Work out the finished part from the listing and answer in its coordinate system (mm). A direction names the side the tool comes from. Give positions to 0.01 mm unless a question says otherwise; leave off trailing zeros. Write each loop counter-clockwise with the first axis right and the second up, starting at its lowest first coordinate (ties: lowest second). Pieces come first, ordered by that corner, then holes. Notation, with made-up numbers: (-19.75, 75) -> (-8.75, 75) arc R11 ccw to (-8.75, 91) -> close; hole circle Ø2 at (12, -15.75). An arc over 180 degrees is marked (long way). Use a Markdown table: item, result. Add a question column.
Q1. Consider line 1 (Y direction, x = 0, z = 3.5); line 2 (Y direction, x = -1.2, z = 2.75). Determine where each line is inside the solid, lowest interval first.
Q2. Section D-D, the plane z = 2.25 is taken. Give the vertices of the cut face in (x, y).
Q3. Section B-B, the plane x = -1.35 is taken. Give the vertices of the cut face in (y, z).
Q4. For faces 5 (the face through (-2, 2, 6.5)), 6 (the face through (2, -2, 6.5)), 7 (the face through (-0.54, 2.44, 9.49)), 8 (the face through (-2, -2, 8.5)), determine the directions among +Z, -Z, +X, -X, +Y, -Y from which every point of the face is accessible in a straight line to the end or side of a thin tool.
Q5. Section C-C, the plane z = 7.75 is taken. Give the vertices of the cut face in (x, y).
Q6. For a pull along Y with two mould halves and no side action, classify faces 1 (the face through (0, -2.5, 8)), 2 (the face through (-2, -2, 6.5)), 3 (the face through (-0.54, 2.44, 3.2)), 4 (the face through (-0.07, 1.5, 5.18)) as pulls with the +Y half, pulls with the -Y half, needs draft (parallel to the pull), parting line crosses it, or undercut.
Q7. This flat-tipped pin is pushed along its axis until it touches: pin 1 Ø2.5 at (x, y) = (0, 0) entering from -Z. Where does it stop, or does it pass through?
Q8. Section A-A, the plane y = 0.85 is taken. Give the vertices of the cut face in (x, z), plus the area to 3 significant figures.
Autodesk Inventor part; units mm, degrees
ref_plane "Arbeitsebene1" through (0, 0, 8.5) normal (0, 0, -1) x (-1, 0, 0)
ref_plane "YZ Plane" through (0, 0, 0) normal (1, 0, 0) x (0, 1, 0)
ref_plane "XZ Plane" through (0, 0, 0) normal (0, 1, 0) x (-1, 0, 0)
sketch "Skizze1" plane through (0, 0, 0) normal (0, 0, 1) x (1, 0, 0)
  circle A0 centre (0, 0) radius 2.5
  dimension "d1" = 5
extrude "Extrusion1" add sketch "Skizze1" along normal blind 10.5
thread "Gewinde1"
sketch "Skizze2" plane through (0, 0, 10.5) normal (0, 0, 1) x (1, 0, 0)
  circle A0 centre (0, 0) radius 1.5
ref_plane "Arbeitsebene1" through (0, 0, 8.5) normal (0, 0, -1) x (-1, 0, 0)
sketch "Skizze3" plane through (0, 0, 8.5) normal (0, 0, -1) x (-1, 0, 0)
  line L0 (-2.5, -2.5) -> (2.5, -2.5)
  line L1 (2.5, -2.5) -> (2.5, 2.5)
  line L2 (2.5, 2.5) -> (-2.5, 2.5)
  line L3 (-2.5, 2.5) -> (-2.5, -2.5)
  line L4 (-2.5, -2.5) -> (2.5, 2.5) construction
  line L5 (2.5, -2.5) -> (-2.5, 2.5) construction
  point P0 (0, 0)
extrude "Extrusion3" add sketch "Skizze3" along normal blind 2
fillet "Rundung2" radius 0.5 4 edges at (2.5, -2.5, 7.5) (2.5, 2.5, 7.5) (-2.5, -2.5, 7.5) (-2.5, 2.5, 7.5)
hole "Bohrung2" at (0, 0, 10.5) direction (0, 0, -1) diameter 3 end through all
properties part number "RadAdapterSchaft"
Result set:
| question | item | result |
|---|---|---|
| 1 | line 1 | y = -2.5 to -1.5, 1.5 to 2.5 |
| 1 | line 2 | y = -2.19 to -0.9, 0.9 to 2.19 |
| 2 | outline | circle Ø5 at (0, 0); hole circle Ø3 at (0, 0) |
| 3 | outline | (-2.5, 6.5) -> (-2.1, 6.5) -> (-2.1, 0) -> (-0.65, 0) -> (-0.65, 10.5) -> (-2.1, 10.5) -> (-2.1, 8.5) -> (-2.5, 8.5) -> close; (0.65, 0) -> (2.1, 0) -> (2.1, 6.5) -> (2.5, 6.5) -> (2.5, 8.5) -> (2.1, 8.5) -> (2.1, 10.5) -> (0.65, 10.5) -> close |
| 4 | face 5 | -Z, -X, +Y |
| 4 | face 6 | -Z, +X, -Y |
| 4 | face 7 | +Z |
| 4 | face 8 | +Z, -X, -Y |
| 5 | outline | (-2.5, -2) arc R0.5 ccw to (-2, -2.5) -> (2, -2.5) arc R0.5 ccw to (2.5, -2) -> (2.5, 2) arc R0.5 ccw to (2, 2.5) -> (-2, 2.5) arc R0.5 ccw to (-2.5, 2) -> close; hole circle Ø3 at (0, 0) |
| 6 | face 1 | pulls with the -Y half |
| 6 | face 2 | needs draft |
| 6 | face 3 | parting line crosses it |
| 6 | face 4 | undercut |
| 7 | pin 1 | passes through |
| 8 | outline | (-2.5, 6.5) -> (-2.35, 6.5) -> (-2.35, 0) -> (-1.24, 0) -> (-1.24, 10.5) -> (-2.35, 10.5) -> (-2.35, 8.5) -> (-2.5, 8.5) -> close; (1.24, 0) -> (2.35, 0) -> (2.35, 6.5) -> (2.5, 6.5) -> (2.5, 8.5) -> (2.35, 8.5) -> (2.35, 10.5) -> (1.24, 10.5) -> close |
| 8 | area | 24.0 mm2 |
